Read the model definition and answer for the solid it produces. Units are mm, in the model's axes. Coordinates: 2 decimals unless noted, no trailing zeros. Write each loop counter-clockwise with the first axis right and the second up, starting at its lowest first coordinate (ties: lowest second). Pieces come first, ordered by that corner, then holes. Notation, with made-up numbers: (32.5, 37) -> (69.5, 37) arc R13 ccw to (69.5, 48) -> close; hole circle Ø2 at (-31, 15). An arc over 180 degrees is marked (long way). One line per item, written item: value. Start each with the question number.
1. Find section B-B, the plane y = 46. Write down the section's boundary in (x, z).
2. Find section C-C, the plane z = 0.6. State how many separate pieces and enclosed holes the cut face has, and give its area (3 significant figures).
3. Given P1, Ø3, axis at x = -4, y = -0.5, coming from the +Z side; P2, Ø0.6, axis at x = -52.5, z = 1, coming from the -Y side, each flat-ended and moving along its own axis, determine where each tip first touches the part or whether it passes through.
4. Find section A-A, the plane y = -15. Write down the section's boundary in (x, z).
5. Consider line 1 along X through (y, z) = (62, 0.3); line 2 along Y through (x, z) = (-23, 0.3); line 3 along Y through (x, z) = (-8.5, 1). Determine where each line is inside the solid, lowest interval first.
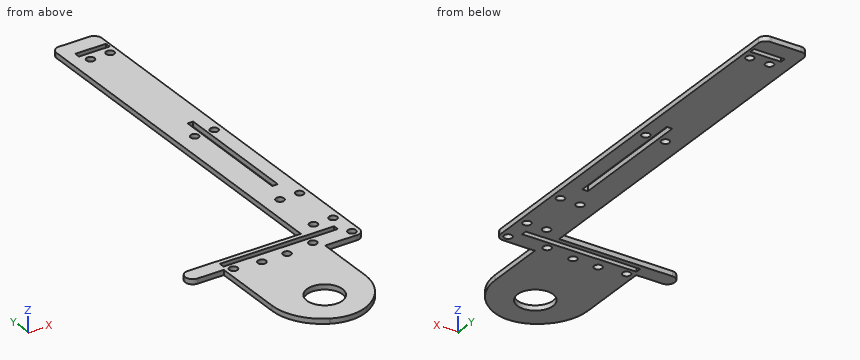
```python
from build123d import *

# Parameters (mm, degrees)
SKETCH_1_R          = 1.6
SKETCH_1_R_2        = 7.08
SKETCH_1_W          = 45.5
SKETCH_1_H          = 2.2
SKETCH_1_W_2        = 2.2
SKETCH_1_H_2        = 50.5
SKETCH_1_W_3        = 12.2
EXTRUDE_1_DEPTH     = 2
SKETCH_2_W          = 4
SKETCH_2_H          = 160
CUT_EXTRUDE_1_DEPTH = 10
SKETCH_3_R          = 1.6
CUT_EXTRUDE_2_DEPTH = 10
FILLET_1_R          = 3


with BuildPart() as part:
    # 草图1 → 凸台-拉伸1 (new body)
    with BuildSketch(Plane.XY):
        with BuildLine():
            Line((-8.65326359, -109.246690295), (-8.65326359, -85.5))
            Line((-8.65326359, -85.5), (11, -85.5))
            Line((11, -85.5), (11, 74.5))
            Line((11, 74.5), (-11, 74.5))
            Line((-11, 74.5), (-11, -74.5))
            Line((-11, -74.5), (-59, -74.5))
            Line((-59, -74.5), (-59, -80.5))
            Line((-59, -80.5), (-45.65326359, -80.5))
            Line((-45.65326359, -80.5), (-45.65326359, -109.246690295))
            ThreePointArc((-45.65326359, -109.246690295), (-42.686252119, -119.728927736), (-34.665533413, -127.101073304))
            Line((-34.665533413, -127.101073304), (-34.351105887, -127.259785353))
            ThreePointArc((-34.351105887, -127.259785353), (-27.15326359, -128.973428312), (-19.955421292, -127.259785353))
            Line((-19.955421292, -127.259785353), (-19.640993767, -127.101073304))
            ThreePointArc((-19.640993767, -127.101073304), (-11.620275061, -119.728927736), (-8.65326359, -109.246690295))
        make_face()
        with Locations((-11, -81.629391896)):
            Circle(SKETCH_1_R, mode=Mode.SUBTRACT)
        with Locations((-42.570682945, -81.629391896)):
            Circle(SKETCH_1_R, mode=Mode.SUBTRACT)
        with Locations((-22.15326359, -83)):
            Circle(SKETCH_1_R, mode=Mode.SUBTRACT)
        with Locations((-27.15326359, -113)):
            Circle(SKETCH_1_R_2, mode=Mode.SUBTRACT)
        with Locations((-32.15326359, -83)):
            Circle(SKETCH_1_R, mode=Mode.SUBTRACT)
        with Locations((-21.75, -77.5)):
            Rectangle(SKETCH_1_W, SKETCH_1_H, mode=Mode.SUBTRACT)
        with Locations((3.8, 61.7)):
            Circle(SKETCH_1_R, mode=Mode.SUBTRACT)
        with Locations((-4, -71.5)):
            Circle(SKETCH_1_R, mode=Mode.SUBTRACT)
        with Locations((3.8, -71.5)):
            Circle(SKETCH_1_R, mode=Mode.SUBTRACT)
        with Locations((-4, -51.5)):
            Circle(SKETCH_1_R, mode=Mode.SUBTRACT)
        with Locations((3.8, -51.5)):
            Circle(SKETCH_1_R, mode=Mode.SUBTRACT)
        with Locations((0, -17.25)):
            Rectangle(SKETCH_1_W_2, SKETCH_1_H_2, mode=Mode.SUBTRACT)
        with Locations((-4, -0.5)):
            Circle(SKETCH_1_R, mode=Mode.SUBTRACT)
        with Locations((3.8, -0.5)):
            Circle(SKETCH_1_R, mode=Mode.SUBTRACT)
        with Locations((-4, 61.7)):
            Circle(SKETCH_1_R, mode=Mode.SUBTRACT)
        with Locations((-0.1, 66.4)):
            Rectangle(SKETCH_1_W_3, SKETCH_1_H, mode=Mode.SUBTRACT)
    extrude(amount=EXTRUDE_1_DEPTH)

    # 草图2 → 切除-拉伸1 (cut)
    with BuildSketch(Plane(origin=(0, 0, 0), x_dir=(-1, 0, 0), z_dir=(0, 0, -1))):
        with Locations((-9, -5.5)):
            Rectangle(SKETCH_2_W, SKETCH_2_H)
    extrude(amount=-CUT_EXTRUDE_1_DEPTH, mode=Mode.SUBTRACT)

    # 草图3 → 切除-拉伸2 (cut)
    with BuildSketch(Plane(origin=(0, 0, 0), x_dir=(-1, 0, 0), z_dir=(0, 0, -1))):
        with Locations((-4, -82.5)):
            Circle(SKETCH_3_R)
    extrude(amount=-CUT_EXTRUDE_2_DEPTH, mode=Mode.SUBTRACT)

    # 圆角1
    fillet_1_edges = [part.edges().sort_by_distance(p)[0] for p in [
        (-59, -74.5, 1),
        (-59, -80.5, 1),
        (7, -85.5, 1),
        (-11, 74.5, 1),
        (7, 74.5, 1),
    ]]
    fillet(fillet_1_edges, radius=FILLET_1_R - 0.0001)  # a hair under: the kernel refuses the full size


solid = part.part
```
Answer block:
1. outline: (-11, 0) -> (7, 0) -> (7, 2) -> (-11, 2) -> close
2. separate pieces: 1
2. enclosed holes: 17
2. area: 4,280 mm2
3. P1: passes through
3. P2: stops at y = -80.5
4. outline: (-11, 0) -> (-1.1, 0) -> (-1.1, 2) -> (-11, 2) -> close; (1.1, 0) -> (7, 0) -> (7, 2) -> (1.1, 2) -> close
5. line 1: x = -11 to -5.57, -2.43 to 2.23, 5.37 to 7
5. line 2: y = -128.42 to -118.73, -107.27 to -84.36, -81.64 to -78.6, -76.4 to -74.5
5. line 3: y = -85.5 to -78.6, -76.4 to 74.46
